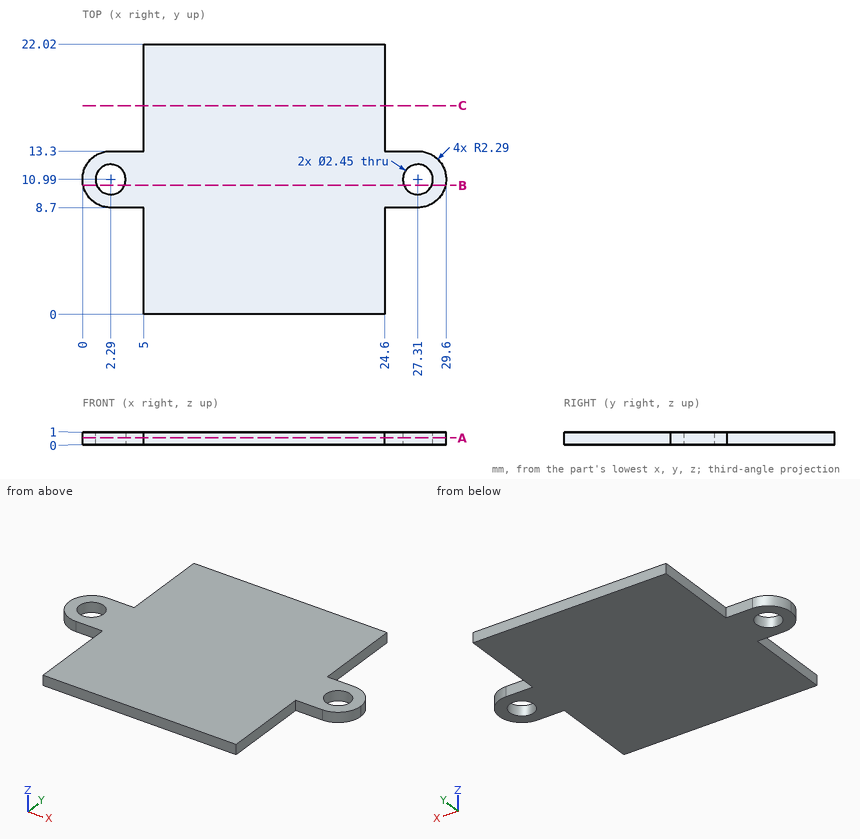
Input: dimensioned drawing with shaded views. Units: mm. Origin: part minimum x, y, z. Give positions to 0.01 mm unless a question says otherwise; leave off trailing zeros. Write each loop counter-clockwise with the first axis right and the second up, starting at its lowest first coordinate (ties: lowest second). Pieces come first, ordered by that corner, then holes.
1. Line query: probe 1 along Y at (x, z) = (2.29, 0.75) (3 decimals); probe 2 along X at (y, z) = (5.5, 0.7); probe 3 along Y at (x, z) = (26.75, 0.5). Output: solid intervals per line, ascending.
2. Section query B-B, the plane y = 10.5. Return loops of the section in (x, z).
3. Section query A-A, the plane z = 0.55. Return loops of the section in (x, y) (3 decimals).
4. Pin query (flat end, axial travel): P1, Ø1.5, axis at x = 27.31, y = 10.99, coming from the +Z side; P2, Ø0.5, axis at y = 18.5, z = 0.5, coming from the +X side. Return the tip coordinate at first contact, or that it passes through.
5. Section query C-C, the plane y = 17. Return loops of the section in (x, z), then the cut area to 3 significant figures.
Computed:
1. probe 1: y = 8.7 to 9.765, 12.215 to 13.3
1. probe 2: x = 5 to 24.6
1. probe 3: y = 8.7 to 9.9, 12.08 to 13.3
2. outline: (0.05, 0) - (1.17, 0) - (1.17, 1) - (0.05, 1) - close; (3.41, 0) - (26.19, 0) - (26.19, 1) - (3.41, 1) - close; (28.43, 0) - (29.55, 0) - (29.55, 1) - (28.43, 1) - close
3. outline: (0, 10.99) arc R2.29 ccw to (2.29, 8.7) - (5, 8.7) - (5, 0) - (24.6, 0) - (24.6, 8.7) - (27.31, 8.7) arc R2.29 ccw to (29.6, 10.99) - (29.6, 11.01) arc R2.29 ccw to (27.31, 13.3) - (24.6, 13.3) - (24.6, 22.02) - (5, 22.02) - (5, 13.3) - (2.29, 13.3) arc R2.29 ccw to (0, 11.01) - close; hole circle Ø2.45 at (2.29, 10.99); hole circle Ø2.45 at (27.31, 10.99)
4. P1: passes through
4. P2: stops at x = 24.6
5. outline: (5, 0) - (24.6, 0) - (24.6, 1) - (5, 1) - close
5. area: 19.6 mm2
